The model under review builds one solid part; all positions refer to its coordinate system, in mm. A direction names the side the tool comes from. Round coordinates to 2 decimals unless told otherwise and drop trailing zeros. Order: outer loops, then holes, each group sorted by start corner. A loop starts at its lowest first (then second) coordinate and runs counter-clockwise, first axis right, second up.
1) To check wall thickness, follow L1, parallel to Y at x = 16.5, z = 12; L2, parallel to Y at x = -3, z = 144. State the ranges of each line that lie inside material, in increasing order.
2) Clearance check with a flat-ended pin moving along its axis: P1, Ø6.5, axis at y = 0, z = 12, coming from the +X side. State where the tip first meets the part, or that it passes through.
3) Machinability: for faces 1 (the face through (15, -6, 7)), 2 (the face through (14, 0, 192)), 3 (the face through (0, 20, 99)), which of the approach directions +Z, -Z, +X, -X, +Y, -Y give a long, thin tool a straight path to every point of the face, cutting with its end or side? Answer none if there is none.
4) Consider section A-A (y = 0). Give the number of separate pieces and of enclosed holes in the cut face, then the cut area to 3 significant figures.
5) Consider section B-B (z = 186). Give the boundary of the cut face in (x, y), then the cut area to 3 significant figures.
6) Mouldability with a two-part tool opening along Z and no side actions: class faces 4 (the face through (-14, 0, 192)), 5 (the face through (15, 0, 18)) as pulls with the +Z half, pulls with the -Z half, needs draft (parallel to the pull), parting line crosses it, or undercut.
Autodesk Fusion 360 part; units mm, degrees
sketch "Sketch1" plane through (0, 0, 0) normal (0, 0, 1) x (1, 0, 0)
  line L0 (20, -20) -> (-20, -20)
  line L1 (-20, -20) -> (-20, 20)
  line L2 (-20, 20) -> (20, 20)
  line L3 (20, 20) -> (20, -20)
  line L4 (20, -20) -> (-20, 20) construction
  line L5 (-20, -20) -> (20, 20) construction
  line L6 (-17, -17) -> (-17, 17)
  line L7 (-17, 17) -> (17, 17)
  line L8 (17, 17) -> (17, -17)
  line L9 (17, -17) -> (-17, -17)
  line L10 (-14, -14) -> (-14, 14)
  line L11 (-14, 14) -> (14, 14)
  line L12 (14, 14) -> (14, -14)
  line L13 (14, -14) -> (-14, -14)
  dimension "d1" = 40
  dimension "d2" = 40
  dimension "d3" = 3
  dimension "d4" = 6
extrude "Extrude1" add sketch "Sketch1" along normal blind 200 contours L0 L1 L2 L3 makes body 1
extrude "Extrude2" add sketch "Sketch1" along normal blind 27 draft -0.1 from surface at 200 separate body contours L6 L7 L8 L9 makes body 2
extrude "Extrude3" add 1 faces at (4.6667, -16, 200) along direction (0, 0, -1) blind 20 on bodies 2 bodies 1 2
chamfer "Chamfer1" distance 3 angle 45 4 edges at (0, 14, 180) (-14, 0, 180) (0, -14, 180) (14, 0, 180) on bodies 1
extrude "Extrude4" add sketch "Sketch1" along normal blind 2 contours L6 L7 L8 L9 | L10 L11 L12 L13 bodies 1
sketch "Sketch2" plane through (20, 0, 0) normal (1, 0, 0) x (0, 1, 0)
  line L0 (-20, 0) -> (20, 0)
  line L1 (20, 0) -> (20, 200)
  line L2 (20, 200) -> (-20, 200)
  line L3 (-20, 200) -> (-20, 0)
  circle A0 centre (0, 12) radius 4
  circle A1 centre (0, 12) radius 6
  line L4 (-6, 12) -> (-6, -0.3727)
  line L5 (6, 12) -> (6, 0)
  dimension "d15" = 8
  dimension "d16" = 12
  dimension "d17" = 2
extrude "Extrude5" add sketch "Sketch2" against normal blind 7 contours L0 A1 L4 L5 | A1 | A0 bodies 1
mirror "Mirror1" about plane through (0, 0, 0) normal (1, 0, 0) of "Extrude5"
hole "Hole1" at (20, 0, 12) direction (-1, 0, 0) diameter 8 end up to surface (40 mm away) bodies 1
Answer below:
1. L1: y = -20 to -17, -6 to -4, 4 to 6, 17 to 20
1. L2: y = -20 to -17, 17 to 20
2. P1: passes through
3. face 1: none
3. face 2: +Z
3. face 3: +Z, -Z, +X, -X, +Y
4. separate pieces: 3
4. enclosed holes: 0
4. area: 1,550 mm2
5. outline: (-20, -20) - (20, -20) - (20, 20) - (-20, 20) - close; hole (-14, -14) - (14, -14) - (14, 14) - (-14, 14) - close
5. area: 816 mm2
6. face 4: needs draft
6. face 5: undercut
